```python
from build123d import *

# Parameters (mm, degrees)
F0_W     = 114
F0_H     = 114
F0_W_2   = 6
F0_H_2   = 6
F0_R     = 1.5
F1_DEPTH = 42
F0_R_2   = 3.5
F2_DEPTH = 38
F0_W_3   = 10
F0_H_3   = 8.5
F3_DEPTH = 2
F4_DEPTH = 2
F5_R     = 3


with BuildPart() as f1:
    # F0 (on Top) → F1 (new body)
    with BuildSketch(Plane.XY):
        Rectangle(F0_W, F0_H)
        Polygon((49, 55), (55, 55), (55, 49), (55, -49), (55, -55), (49, -55), (46, -55), (36, -55), (24, -55), (14, -55), (11, -55), (-11, -55), (-14, -55), (-24, -55), (-36, -55), (-46, -55), (-49, -55), (-55, -55), (-55, -49), (-55, 49), (-55, 55), (-49, 55), (-46, 55), (-36, 55), (-24, 55), (-14, 55), (-11, 55), (11, 55), (14, 55), (24, 55), (36, 55), (46, 55), align=None, mode=Mode.SUBTRACT)
        Polygon((-11, 40), (-11, 55), (-14, 55), (-14, 46.5), (-14, 40), align=None)
        Polygon((14, 46.5), (14, 55), (11, 55), (11, 40), (14, 40), align=None)
        Polygon((49, 49), (49, 55), (46, 55), (46, 46.5), (46, 40), (49, 40), align=None)
        Polygon((-46, 46.5), (-46, 55), (-49, 55), (-49, 49), (-49, 40), (-46, 40), align=None)
        Polygon((-49, -55), (-46, -55), (-46, -46.5), (-46, -40), (-49, -40), (-49, -49), align=None)
        Polygon((-14, -55), (-11, -55), (-11, -40), (-14, -40), (-14, -46.5), align=None)
        Polygon((11, -55), (14, -55), (14, -46.5), (14, -40), (11, -40), align=None)
        Polygon((49, -55), (49, -49), (49, -40), (46, -40), (46, -46.5), (46, -55), align=None)
        with Locations((-52, 52)):
            Rectangle(F0_W_2, F0_H_2)
        with Locations((-52, 52)):
            Circle(F0_R, mode=Mode.SUBTRACT)
        with Locations((52, 52)):
            Rectangle(F0_W_2, F0_H_2)
        with Locations((52, 52)):
            Circle(F0_R, mode=Mode.SUBTRACT)
        with Locations((52, -52)):
            Rectangle(F0_W_2, F0_H_2)
        with Locations((52, -52)):
            Circle(F0_R, mode=Mode.SUBTRACT)
        with Locations((-52, -52)):
            Rectangle(F0_W_2, F0_H_2)
        with Locations((-52, -52)):
            Circle(F0_R, mode=Mode.SUBTRACT)
    extrude(amount=F1_DEPTH)

    # F0 (on Top) → F2, piece 5 (join)
    with BuildSketch(Plane.XY):
        with Locations((-41, 50.75)):
            Rectangle(F0_W_3, F0_H_3)
        with Locations((-19, 50.75)):
            Rectangle(F0_W_3, F0_H_3)
        with Locations((19, 50.75)):
            Rectangle(F0_W_3, F0_H_3)
        with Locations((41, 50.75)):
            Rectangle(F0_W_3, F0_H_3)
        with Locations((-19, -50.75)):
            Rectangle(F0_W_3, F0_H_3)
        with Locations((-41, -50.75)):
            Rectangle(F0_W_3, F0_H_3)
        with Locations((19, -50.75)):
            Rectangle(F0_W_3, F0_H_3)
        with Locations((41, -50.75)):
            Rectangle(F0_W_3, F0_H_3)
    extrude(amount=F2_DEPTH)

    # F0 (on Top) → F3 (join)
    with BuildSketch(Plane.XY):
        with Locations((52, 52)):
            Rectangle(F0_W_2, F0_H_2)
        with Locations((52, 52)):
            Circle(F0_R, mode=Mode.SUBTRACT)
        with Locations((52, -52)):
            Rectangle(F0_W_2, F0_H_2)
        with Locations((52, -52)):
            Circle(F0_R, mode=Mode.SUBTRACT)
    extrude(amount=F3_DEPTH)



with BuildPart() as f2:
    # F0 (on Top) → F2 (new body)
    with BuildSketch(Plane.XY):
        with Locations((-30, 41.5)):
            Circle(F0_R_2)
        with Locations((-30, 41.5)):
            Circle(F0_R, mode=Mode.SUBTRACT)
    extrude(amount=F2_DEPTH)


with BuildPart() as f2b:
    # F0 (on Top) → F2, piece 2 (new body)
    with BuildSketch(Plane.XY):
        with Locations((30, 41.5)):
            Circle(F0_R_2)
        with Locations((30, 41.5)):
            Circle(F0_R, mode=Mode.SUBTRACT)
    extrude(amount=F2_DEPTH)


with BuildPart() as f2c:
    # F0 (on Top) → F2, piece 3 (new body)
    with BuildSketch(Plane.XY):
        with Locations((30, -41.5)):
            Circle(F0_R_2)
        with Locations((30, -41.5)):
            Circle(F0_R, mode=Mode.SUBTRACT)
    extrude(amount=F2_DEPTH)


with BuildPart() as f2d:
    # F0 (on Top) → F2, piece 4 (new body)
    with BuildSketch(Plane.XY):
        with Locations((-30, -41.5)):
            Circle(F0_R_2)
        with Locations((-30, -41.5)):
            Circle(F0_R, mode=Mode.SUBTRACT)
    extrude(amount=F2_DEPTH)


with BuildPart() as f1_1:
    add(f1.part)

    add(f2.part)  # F4 merges F2

    add(f2b.part)  # F4 merges F2b

    add(f2c.part)  # F4 merges F2c

    add(f2d.part)  # F4 merges F2d
    # F0 (on Top) → F4 (join)
    with BuildSketch(Plane.XY):
        Polygon((55, -49), (55, 49), (49, 49), (49, 40), (46, 40), (46, 46.5), (36, 46.5), (36, 55), (24, 55), (24, 46.5), (14, 46.5), (14, 40), (11, 40), (11, 55), (-11, 55), (-11, 40), (-14, 40), (-14, 46.5), (-24, 46.5), (-24, 55), (-36, 55), (-36, 46.5), (-46, 46.5), (-46, 40), (-49, 40), (-49, 49), (-55, 49), (-55, -49), (-49, -49), (-49, -40), (-46, -40), (-46, -46.5), (-36, -46.5), (-36, -55), (-24, -55), (-24, -46.5), (-14, -46.5), (-14, -40), (-11, -40), (-11, -55), (11, -55), (11, -40), (14, -40), (14, -46.5), (24, -46.5), (24, -55), (36, -55), (36, -46.5), (46, -46.5), (46, -40), (49, -40), (49, -49), align=None)
        with Locations((-30, -41.5)):
            Circle(F0_R_2, mode=Mode.SUBTRACT)
        with Locations((30, -41.5)):
            Circle(F0_R_2, mode=Mode.SUBTRACT)
        with Locations((-30, 41.5)):
            Circle(F0_R_2, mode=Mode.SUBTRACT)
        with Locations((30, 41.5)):
            Circle(F0_R_2, mode=Mode.SUBTRACT)
        with Locations((-52, 52)):
            Circle(F0_R)
        with Locations((-30, 41.5)):
            Circle(F0_R)
        with Locations((30, 41.5)):
            Circle(F0_R)
        with Locations((52, 52)):
            Circle(F0_R)
        with Locations((-52, -52)):
            Circle(F0_R)
        with Locations((-30, -41.5)):
            Circle(F0_R)
        with Locations((30, -41.5)):
            Circle(F0_R)
        with Locations((52, -52)):
            Circle(F0_R)
    extrude(amount=F4_DEPTH)

    # F5
    f5_edges = [f1_1.edges().sort_by_distance(p)[0] for p in [
        (-57, 57, 21),
        (57, 57, 21),
        (-57, -57, 21),
        (57, -57, 21),
    ]]
    fillet(f5_edges, radius=F5_R)


solid = f1_1.part
```
For this review, take the finished solid that the model builds, in its own axes (mm). Coordinates: 2 decimals unless noted, no trailing zeros. Loops run counter-clockwise (first coordinate to the right, second up) from the corner with the lowest first, then second, coordinate; pieces in that order, holes last.
1. Add section D-D, the plane x = 30. Give the boundary of the cut face in (y, z).
2. For line 1 (Y direction, x = -52, z = 18); line 2 (Y direction, x = -40.5, z = 5); line 3 (Y direction, x = -8, z = 22), list the stretches that pass through material, from the lowest coordinate up.
3. Mouldability with a two-part tool opening along Y and no side actions: class faces 1 (the flat face through (47, 40, 22)), 2 (the cylindrical face through (-56.14, -56.1, 21.29)) as +Y half, -Y half, draft (parallel to the pull), parting line (faces both ways), or undercut.
4. Add section B-B, the plane z = 3.5. Count the separate pieces of the cut face and the enclosed holes in it, then the cut area to 3 significant figures.
5. Insertion check: P1, Ø6, axis at x = -16.5, y = 38, coming from the +Z side; P2, Ø10, axis at x = -29.5, y = 32, coming from the -Z side; P3, Ø7, axis at x = 18, y = 50.5, coming from the +Z side. Each pin has a flat end and moves straight along its axis. Give the tip position at first contact, or say it passes through.
6. Add section A-A, the plane x = -52. Give the boundary of the cut face in (y, z).
Result:
1. outline: (-57, 0) - (57, 0) - (57, 42) - (55, 42) - (55, 2) - (45, 2) - (45, 38) - (43, 38) - (43, 2) - (40, 2) - (40, 38) - (38, 38) - (38, 2) - (-38, 2) - (-38, 38) - (-40, 38) - (-40, 2) - (-43, 2) - (-43, 38) - (-45, 38) - (-45, 2) - (-55, 2) - (-55, 42) - (-57, 42) - close
2. line 1: y = -57 to -53.5, -50.5 to -49, 49 to 50.5, 53.5 to 57
2. line 2: y = -57 to -46.5, 46.5 to 57
2. line 3: y = -57 to -55, 55 to 57
3. face 1: undercut
3. face 2: -Y half
4. separate pieces: 5
4. enclosed holes: 9
4. area: 2,170 mm2
5. P1: stops at z = 2
5. P2: stops at z = 0
5. P3: stops at z = 38
6. outline: (-57, 0) - (57, 0) - (57, 42) - (53.5, 42) - (53.5, 2) - (50.5, 2) - (50.5, 42) - (49, 42) - (49, 2) - (-49, 2) - (-49, 42) - (-50.5, 42) - (-50.5, 2) - (-53.5, 2) - (-53.5, 42) - (-57, 42) - close
